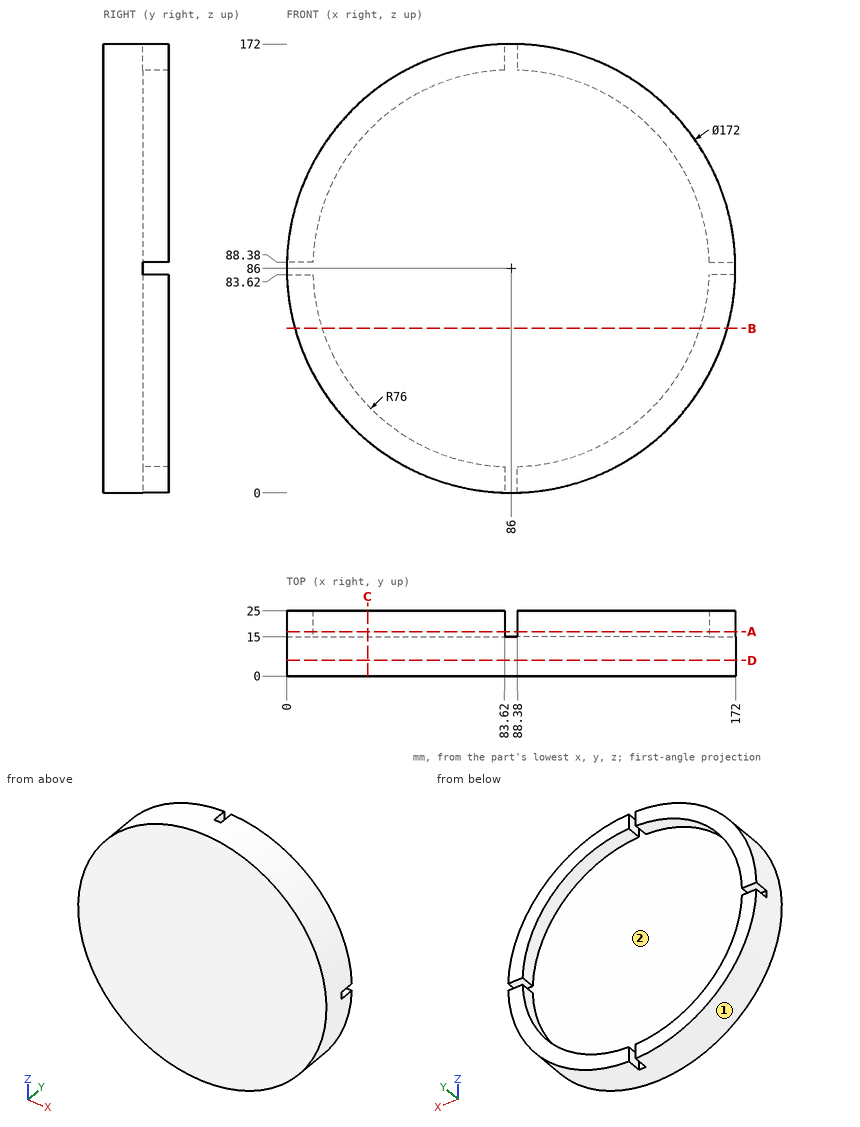
For this review, use the dimensioned drawing (mm, ordinates from the lowest corner) and the shaded views. A direction names the side the tool comes from. Coordinates: 2 decimals unless noted, no trailing zeros. Loops run counter-clockwise (first coordinate to the right, second up) from the corner with the lowest first, then second, coordinate; pieces in that order, holes last. Notation, with made-up numbers: M 38.5,45 L 54.5,45 A10 cw 54.5,50 Z; hole C 39.25,-18 d10. An arc over 180 degrees is marked long. Answer as CSV lines item,"result".
Item 1: For probe 1 along Y at (x, z) = (76.5, 139); probe 2 along X at (y, z) = (23.75, 104); probe 3 along Z at (x, y) = (21, 19.5), list the stretches that pass through material, from the lowest coordinate up.
Answer list:
probe 1,"0 to 15"
probe 2,"1.9 to 12.16, 159.84 to 170.1"
probe 3,"29.69 to 46.62, 125.38 to 142.31"
Item 2: Add section B-B on z = 63. State the section outline as (x, y) points, plus the area to 3 significant figures.
Answer list:
outline,"M 3.13,0 L 168.87,0 L 168.87,25 L 158.44,25 L 158.44,15 L 13.56,15 L 13.56,25 L 3.13,25 Z"
area,"2,690 mm²"
Item 3: For P1, Ø11, axis at y = 22, z = 7, coming from the +X side; P2, Ø3, axis at y = 19, z = 165.5, coming from the +X side; P3, Ø11, axis at x = 165.5, y = 19, coming from the -Z side, all flat-tipped, find the tip position at first contact; note any pin that passes through.
Answer list:
P1,"x = 130.65"
P2,"x = 122.22"
P3,"z = 42.18"
Item 4: Add section D-D on y = 6. State the section outline as (x, z) points, plus the area to 3 significant figures.
Answer list:
outline,"C 86,86 d172"
area,"23,200 mm²"
Item 5: Machinability: for the marked faces 1 and 2, which of the approach directions +Z, -Z, +X, -X, +Y, -Y give a long, thin tool a straight path to every point of the face, cutting with its end or side? Answer none if there is none.
Answer list:
face 1,"+Y, -Y"
face 2,"+Y"
Item 6: Add section C-C on x = 31. State the section outline as (y, z) points.
Answer list:
outline,"M 0,19.89 L 25,19.89 L 25,33.55 L 15,33.55 L 15,138.45 L 25,138.45 L 25,152.11 L 0,152.11 Z"
Item 7: Add section A-A on y = 17. State the section outline as (x, z) points, plus the area to 3 significant figures.
Answer list:
outline,"M 0.03,83.62 A86 ccw 83.62,0.03 L 83.62,10.04 A76 cw 10.04,83.62 Z; M 0.03,88.38 L 10.04,88.38 A76 cw 83.62,161.96 L 83.62,171.97 A86 ccw Z; M 88.38,0.03 A86 ccw 171.97,83.62 L 161.96,83.62 A76 cw 88.38,10.04 Z; M 88.38,161.96 A76 cw 161.96,88.38 L 171.97,88.38 A86 ccw 88.38,171.97 Z"
area,"4,900 mm²"
